Geometry: final body of the model. Coordinates: model frame, mm. A direction names the side the tool comes from. Give positions to 0.01 mm unless a question says otherwise; leave off trailing zeros. Loops run counter-clockwise (first coordinate to the right, second up) from the corner with the lowest first, then second, coordinate; pieces in that order, holes last. Notation, with made-up numbers: (3, 49) - (55, 49) arc R6 cw to (55, 57) - close; hole circle Ø3 at (43.25, 66.5). An arc over 180 degrees is marked (long way). Answer in a Markdown table with one row per item.
from build123d import *

# Parameters (mm, degrees)
IZIM1_W                     = 60
IZIM1_H                     = 40
IZIM1_W_2                   = 30
IZIM1_H_2                   = 2
IZIM1_W_3                   = 8
Y_KSEKLIK_EKSTR_ZYON1_DEPTH = 40
IZIM1_3_W                   = 8
IZIM1_3_H                   = 2
IZIM1_3_W_2                 = 30
Y_KSEKLIK_EKSTR_ZYON2_DEPTH = 20
IZIM4_R                     = 2
KES_EKSTR_ZYON1_DEPTH       = 37
KES_EKSTR_ZYON2_DEPTH       = 20


with BuildPart() as part:
    # izim1 → Y_kseklik-Ekstr_zyon1 (new body)
    with BuildSketch(Plane.XY):
        Rectangle(IZIM1_W, IZIM1_H)
        with Locations((0, -14)):
            Rectangle(IZIM1_W_2, IZIM1_H_2, mode=Mode.SUBTRACT)
        with Locations((24.5, 15)):
            Rectangle(IZIM1_W_3, IZIM1_H_2, mode=Mode.SUBTRACT)
        with Locations((-24.5, 14)):
            Rectangle(IZIM1_W_3, IZIM1_H_2, mode=Mode.SUBTRACT)
        with Locations((-24.5, 14)):
            Rectangle(IZIM1_W_3, IZIM1_H_2)
        with Locations((24.5, 15)):
            Rectangle(IZIM1_W_3, IZIM1_H_2)
        with Locations((0, -14)):
            Rectangle(IZIM1_W_2, IZIM1_H_2)
    extrude(amount=-Y_KSEKLIK_EKSTR_ZYON1_DEPTH)

    # izim1_3 → Y_kseklik-Ekstr_zyon2 (add)
    with BuildSketch(Plane.XY):
        with Locations((-24.5, 14)):
            Rectangle(IZIM1_3_W, IZIM1_3_H)
        with Locations((24.5, 15)):
            Rectangle(IZIM1_3_W, IZIM1_3_H)
        with Locations((0, -14)):
            Rectangle(IZIM1_3_W_2, IZIM1_3_H)
    extrude(amount=Y_KSEKLIK_EKSTR_ZYON2_DEPTH)

    # izim4 → Kes-Ekstr_zyon1 (cut, through all)
    with BuildSketch(Plane(origin=(0, 16, 0), x_dir=(1, 0, 0), z_dir=(0, 1, 0))):
        with Locations((-24.5, -15)):
            Circle(IZIM4_R)
        with Locations((-24.5, -5)):
            Circle(IZIM4_R)
        with Locations((24.5, -5)):
            Circle(IZIM4_R)
        with Locations((24.5, -15)):
            Circle(IZIM4_R)
        with BuildLine():
            ThreePointArc((23.5, -20), (21.378679656, -19.121320344), (20.5, -17))
            Line((20.5, -17), (20.5, -20))
            Line((20.5, -20), (23.5, -20))
        make_face()
        with BuildLine():
            Line((28.5, -20), (28.5, -17))
            ThreePointArc((28.5, -17), (27.621320344, -19.121320344), (25.5, -20))
            Line((25.5, -20), (28.5, -20))
        make_face()
        with BuildLine():
            ThreePointArc((-25.5, -20), (-27.621320344, -19.121320344), (-28.5, -17))
            Line((-28.5, -17), (-28.5, -20))
            Line((-28.5, -20), (-25.5, -20))
        make_face()
        with BuildLine():
            Line((-20.5, -20), (-20.5, -17))
            ThreePointArc((-20.5, -17), (-21.378679656, -19.121320344), (-23.5, -20))
            Line((-23.5, -20), (-20.5, -20))
        make_face()
    extrude(amount=-KES_EKSTR_ZYON1_DEPTH, mode=Mode.SUBTRACT)

    # izim5 → Kes-Ekstr_zyon2 (cut)
    with BuildSketch(Plane.XZ.offset(15)):
        with BuildLine():
            Line((-15, 20), (-15, 15))
            ThreePointArc((-15, 15), (-13.535533906, 18.535533906), (-10, 20))
            Line((-10, 20), (-15, 20))
        make_face()
        with BuildLine():
            Line((15, 20), (10, 20))
            ThreePointArc((10, 20), (13.535533906, 18.535533906), (15, 15))
            Line((15, 15), (15, 20))
        make_face()
    extrude(amount=-KES_EKSTR_ZYON2_DEPTH, mode=Mode.SUBTRACT)


solid = part.part
Q1. Cut plane A-A (x = 24.5). Output: boundary loops of the cut face in (y, z), and give its area (3 significant figures).
Check values:
| item | result |
|---|---|
| outline | (-20, -40) - (20, -40) - (20, 0) - (16, 0) - (16, 3) - (14, 3) - (14, 0) - (-20, 0) - close; (14, 7) - (16, 7) - (16, 13) - (14, 13) - close; (14, 17) - (16, 17) - (16, 20) - (14, 20) - close |
| area | 1,620 mm² |
Q2. Reachability of faces 1 (the flat face through (-25, 13, 10)), 2 (the flat face through (20.5, 15, 8)), 3 (the flat face through (15, -14, 7)), 4 (the flat face through (-28.5, 14, 8)) from +Z, -Z, +X, -X, +Y, -Y: full face, straight path, thin tool, end or side. Return the list, or none.
Check values:
| item | result |
|---|---|
| face 1 | +Z, +X, -X, -Y |
| face 2 | +Z, +Y, -Y |
| face 3 | +Z, +X, +Y, -Y |
| face 4 | +Z, -X, +Y, -Y |
Q3. Cut plane D-D (z = 12). Output: boundary loops of the cut face in (x, y).
Check values:
| item | result |
|---|---|
| outline | (-28.5, 13) - (-20.5, 13) - (-20.5, 15) - (-28.5, 15) - close; (-15, -15) - (15, -15) - (15, -13) - (-15, -13) - close; (20.5, 14) - (28.5, 14) - (28.5, 16) - (20.5, 16) - close |
Q4. Material intervals for line 1 along Z through (x, y) = (24.5, 15.3); line 2 along X through (y, z) = (14.9, 15); line 3 along Z through (x, y) = (-24, 14), sorted ascending.
Check values:
| item | result |
|---|---|
| line 1 | -40 to 3, 7 to 13, 17 to 20 |
| line 2 | -28.5 to -26.5, -22.5 to -20.5, 20.5 to 22.5, 26.5 to 28.5 |
| line 3 | -40 to 3.06, 6.94 to 13.06, 16.94 to 20 |
Q5. Cut plane B-B (z = 5). Output: boundary loops of the cut face in (x, y), and give its area (3 significant figures).
Check values:
| item | result |
|---|---|
| outline | (-28.5, 13) - (-26.5, 13) - (-26.5, 15) - (-28.5, 15) - close; (-22.5, 13) - (-20.5, 13) - (-20.5, 15) - (-22.5, 15) - close; (-15, -15) - (15, -15) - (15, -13) - (-15, -13) - close; (20.5, 14) - (22.5, 14) - (22.5, 16) - (20.5, 16) - close; (26.5, 14) - (28.5, 14) - (28.5, 16) - (26.5, 16) - close |
| area | 76.0 mm² |
Q6. Cut plane C-C (x = 13). Output: boundary loops of the cut face in (y, z).
Check values:
| item | result |
|---|---|
| outline | (-20, -40) - (20, -40) - (20, 0) - (-13, 0) - (-13, 19) - (-15, 19) - (-15, 0) - (-20, 0) - close |
Q7. Draft query along X for faces 5 (the cylindrical face through (-27.6, 14.01, 19.14)), 6 (the flat face through (0, 20, -20)), 7 (the cylindrical face through (-21.36, 14.01, 19.1)). Return one class per face: pulls with the +X half, pulls with the -X half, needs draft (parallel to the pull), parting line crosses it, or undercut.
Check values:
| item | result |
|---|---|
| face 5 | pulls with the -X half |
| face 6 | needs draft |
| face 7 | undercut |
Q8. First-contact query: pin 1 (2.5 mm diameter, centred on x = 23, z = 12.5, fed in from +Y); pin 2 (1 mm diameter, centred on y = 15, z = 11, fed in from +X); pin 3 (6 mm diameter, centred on x = 19, y = -9.5, fed in from +Z); pin 4 (2.5 mm diameter, centred on x = 24.5, z = 15, fed in from +Y). Flat tips, straight axial feed; report the tip coordinate or a pass-through.
Check values:
| item | result |
|---|---|
| pin 1 | y = 16 |
| pin 2 | x = 28.5 |
| pin 3 | z = 0 |
| pin 4 | through |
